```python
from build123d import *

# Parameters (mm, degrees)
CROQUIS2_W              = 30
CROQUIS2_H              = 20
SALIENTE_EXTRUIR2_DEPTH = 25
SALIENTE_EXTRUIR3_DEPTH = 30
REDONDEO1_R             = 5


with BuildPart() as part:
    # Croquis2 → Saliente-Extruir2 (new body)
    with BuildSketch(Plane(origin=(0, 0, 0), x_dir=(0, 0, -1), z_dir=(1, 0, 0))):
        with Locations((-15, -10)):
            Rectangle(CROQUIS2_W, CROQUIS2_H)
    extrude(amount=SALIENTE_EXTRUIR2_DEPTH)

    # Croquis3 → Saliente-Extruir3 (add, through all)
    with BuildSketch(Plane(origin=(0, 0, 0), x_dir=(-1, 0, 0), z_dir=(0, 0, -1))):
        Polygon((0, 0), (0, 25), (-25, 0), align=None)
    extrude(amount=-SALIENTE_EXTRUIR3_DEPTH)

    # Redondeo1
    redondeo1_edges = [part.edges().sort_by_distance(p)[0] for p in [
        (0, 25, 15),
    ]]
    fillet(redondeo1_edges, radius=REDONDEO1_R)


solid = part.part
```
Geometry check sheet. Reference: the model listing, model coordinates, mm. Give positions to 0.01 mm unless a question says otherwise; leave off trailing zeros. Write each loop counter-clockwise with the first axis right and the second up, starting at its lowest first coordinate (ties: lowest second). Pieces come first, ordered by that corner, then holes.
1) Gauge pin test, flat end, axial feed: pin 1 (5 mm diameter, centred on x = 14.5, z = 14, fed in from +Y). Record the tip position at first contact, or that the pin passes through.
2) Section check B-B, the plane z = 12.5. Record the boundary of the cut face in (x, y).
3) Section check A-A, the plane x = 9. Record the boundary of the cut face in (y, z).
4) Material ranges on L1, parallel to Y at x = 5.5, z = 12.25; L2, parallel to X at y = 9.5, z = 10.5; L3, parallel to X at y = 3, z = 11.75, recorded low to high.
5) Section check C-C, the plane y = 5. Record the boundary of the cut face in (x, z).
Computed:
1. pin 1: stops at y = 13
2. outline: (0, -20) - (25, -20) - (25, 0) - (8.54, 16.46) arc R5 ccw to (0, 12.93) - close
3. outline: (-20, 0) - (16, 0) - (16, 30) - (-20, 30) - close
4. L1: y = -20 to 17.9
4. L2: x = 0 to 15.5
4. L3: x = 0 to 22
5. outline: (0, 0) - (20, 0) - (20, 30) - (0, 30) - close
